Study the drawing (mm; zero at the part's minimum x, y, z) and answer. A direction names the side the tool comes from. Coordinates: 2 decimals unless noted, no trailing zeros. Order: outer loops, then holes, each group sorted by start corner. A loop starts at its lowest first (then second) coordinate and runs counter-clockwise, first axis right, second up. Notation, with made-up numbers: (23.25, -14) -> (56.25, -14) arc R22 cw to (56.25, 15) -> close; hole circle Ø5 at (48.5, 20.5). An arc over 180 degrees is marked (long way). Answer in a Markdown table with one row per item. Add a question column.
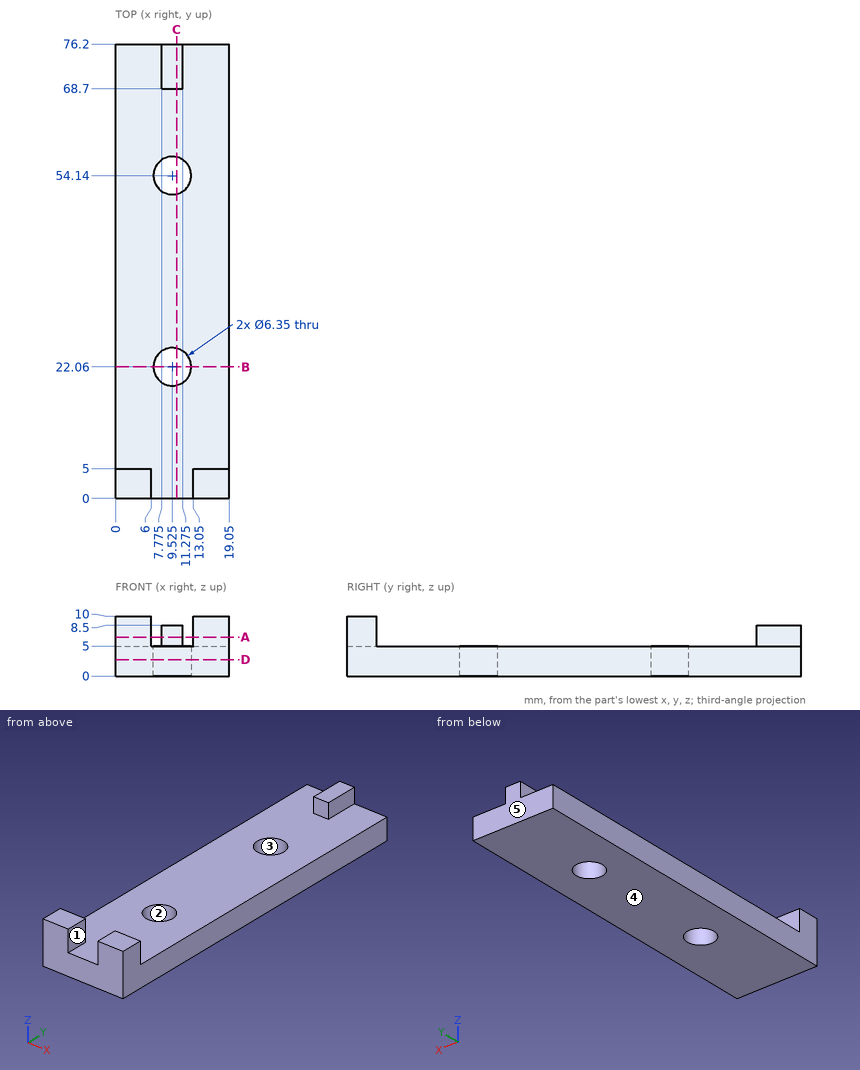
Q1. Straight lines are drawn through the part: line 1 (Y direction, x = 8, z = 3); line 2 (Z direction, x = 1.5, y = 32.5). For each, find the intervals that lie inside material, in ascending order.
Q2. A cutting plane is placed at B-B (y = 22.06). Determine the outline of the cut face in (x, z), then the cut area to 3 significant figures.
Q3. A cutting plane is placed at A-A (z = 6.5). Determine the outline of the cut face in (x, y) (3 decimals), then the cut area to 4 significant figures.
Q4. Determine the mould class of the marked faces 3, 4 and 5 for opening direction Y: +Y half, -Y half, draft (parallel to the pull), parting line (faces both ways), or undercut.
Q5. For the marked faces 1 and 2, determine the directions among +Z, -Z, +X, -X, +Y, -Y from which every point of the face is accessible in a straight line to the end or side of a thin tool.
Q6. A cutting plane is placed at D-D (z = 2.75). Determine the outline of the cut face in (x, y) (3 decimals).
Q7. A cutting plane is placed at C-C (x = 10.25). Determine the outline of the cut face in (y, z), then the cut area to 3 significant figures.
Q8. Given pin 1 (1 mm diameter, centred on x = 9.5, y = 72.5, fed in from +Z); pin 2 (2 mm diameter, centred on x = 17, y = 13, fed in from +Z); pin 3 (3 mm diameter, centred on x = 10, y = 38, fed in from -Z); pin 4 (3 mm diameter, centred on x = 9, z = 7, fed in from -Y), each flat-ended and moving along its own axis, determine where each tip first touches the part or whether it passes through.
Returned:
| question | item | result |
|---|---|---|
| 1 | line 1 | y = 0 to 19.28, 24.84 to 51.36, 56.92 to 76.2 |
| 1 | line 2 | z = 0 to 5 |
| 2 | outline | (0, 0) -> (6.35, 0) -> (6.35, 5) -> (0, 5) -> close; (12.7, 0) -> (19.05, 0) -> (19.05, 5) -> (12.7, 5) -> close |
| 2 | area | 63.5 mm² |
| 3 | outline | (0, 0) -> (6, 0) -> (6, 5) -> (0, 5) -> close; (7.775, 68.7) -> (11.275, 68.7) -> (11.275, 76.2) -> (7.775, 76.2) -> close; (13.05, 0) -> (19.05, 0) -> (19.05, 5) -> (13.05, 5) -> close |
| 3 | area | 86.25 mm² |
| 4 | face 3 | undercut |
| 4 | face 4 | draft |
| 4 | face 5 | +Y half |
| 5 | face 1 | +Z, +Y, -Y |
| 5 | face 2 | +Z, -Z |
| 6 | outline | (0, 0) -> (19.05, 0) -> (19.05, 76.2) -> (0, 76.2) -> close; hole circle Ø6.35 at (9.525, 22.06); hole circle Ø6.35 at (9.525, 54.14) |
| 7 | outline | (0, 0) -> (18.97, 0) -> (18.97, 5) -> (0, 5) -> close; (25.15, 0) -> (51.05, 0) -> (51.05, 5) -> (25.15, 5) -> close; (57.23, 0) -> (76.2, 0) -> (76.2, 8.5) -> (68.7, 8.5) -> (68.7, 5) -> (57.23, 5) -> close |
| 7 | area | 345 mm² |
| 8 | pin 1 | stops at z = 8.5 |
| 8 | pin 2 | stops at z = 5 |
| 8 | pin 3 | stops at z = 0 |
| 8 | pin 4 | stops at y = 68.7 |
